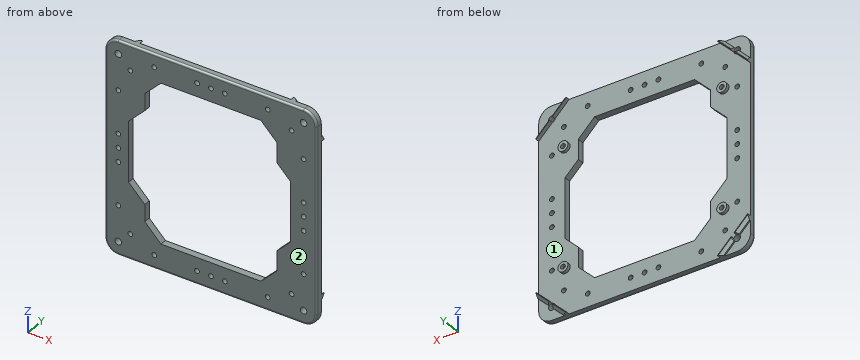
from build123d import *
from build123d.topology import SkipClean

# Parameters (mm, degrees)
SKETCH1_W           = 203.2
SKETCH1_H           = 203.2
BOSS_EXTRUDE1_DEPTH = 6.35
FILLET1_R           = 12.7
SKETCH2_R           = 3.175
CUT_EXTRUDE1_DEPTH  = 288.438345563
FILLET2_R           = 1.905
SKETCH3_R           = 2.286
CUT_EXTRUDE2_DEPTH  = 288.438345634
SKETCH4_R           = 2.286
CUT_EXTRUDE3_DEPTH  = 288.438345634
SKETCH5_R           = 4.826
SKETCH5_R_2         = 2.286
BOSS_EXTRUDE2_DEPTH = 3.175
BOSS_EXTRUDE3_DEPTH = 3.81
CHAMFER1_SIZE       = 2.54
CUT_EXTRUDE4_DEPTH  = 288.438345634
CHAMFER2_SIZE       = 15.5448
SKETCH8_R           = 2.286
CUT_EXTRUDE5_DEPTH  = 288.438345634


with BuildPart() as part:
    # Sketch1 → Boss-Extrude1 (new body)
    with BuildSketch(Plane(origin=(0, 0, 0), x_dir=(1, 0, 0), z_dir=(0, 1, 0))):
        with Locations((101.6, 101.6)):
            Rectangle(SKETCH1_W, SKETCH1_H)
    extrude(amount=BOSS_EXTRUDE1_DEPTH)

    # Fillet1
    fillet1_edges = [part.edges().sort_by_distance(p)[0] for p in [
        (0, 3.175, -203.2),
        (203.2, 3.175, -203.2),
        (203.2, 3.175, 0),
        (0, 3.175, 0),
    ]]
    fillet(fillet1_edges, radius=FILLET1_R)

    # Sketch2 → Cut-Extrude1 (cut, through all)
    with BuildSketch(Plane.XZ):
        with Locations(Location((12.7, -12.7, 0), (0, 0, 270))):
            Circle(SKETCH2_R)
        with Locations(Location((190.5, -12.7, 0), (0, 0, 270))):
            Circle(SKETCH2_R)
        with Locations(Location((190.5, -190.5, 0), (0, 0, 270))):
            Circle(SKETCH2_R)
        with Locations(Location((12.7, -190.5, 0), (0, 0, 270))):
            Circle(SKETCH2_R)
    extrude(amount=-CUT_EXTRUDE1_DEPTH, mode=Mode.SUBTRACT)

    # Fillet2
    fillet2_edges = [part.edges().sort_by_distance(p)[0] for p in [
        (0, 0, -101.6),
        (101.6, 0, -203.2),
        (203.2, 0, -101.6),
        (101.6, 0, 0),
        (199.480256121, 0, -199.480256121),
        (199.480256121, 0, -3.719743879),
        (3.719743879, 0, -3.719743879),
        (3.719743879, 0, -199.480256121),
    ]]
    fillet(fillet2_edges, radius=FILLET2_R)

    # Sketch3 → Cut-Extrude2 (cut, through all)
    with BuildSketch(Plane(origin=(0, 6.35, 0), x_dir=(1, 0, 0), z_dir=(0, 1, 0))):
        with Locations(Location((24.197781122, 24.197781122, 0), (0, 0, 270))):
            Circle(SKETCH3_R)
        with Locations(Location((179.002218878, 179.002218878, 0), (0, 0, 270))):
            Circle(SKETCH3_R)
        with Locations(Location((179.002218878, 24.197781122, 0), (0, 0, 270))):
            Circle(SKETCH3_R)
        with Locations(Location((24.197781122, 179.002218878, 0), (0, 0, 270))):
            Circle(SKETCH3_R)
    extrude(amount=-CUT_EXTRUDE2_DEPTH, mode=Mode.SUBTRACT)

    # Sketch4 → Cut-Extrude3 (cut, through all)
    with BuildSketch(Plane(origin=(0, 6.35, 0), x_dir=(1, 0, 0), z_dir=(0, 1, 0))):
        with Locations(Location((47.117, 12.7, 0), (0, 0, 270))):
            Circle(SKETCH4_R)
        with Locations(Location((156.083, 12.7, 0), (0, 0, 270))):
            Circle(SKETCH4_R)
        with Locations(Location((12.7, 156.083, 0), (0, 0, 270))):
            Circle(SKETCH4_R)
        with Locations(Location((12.7, 47.117, 0), (0, 0, 270))):
            Circle(SKETCH4_R)
        with Locations(Location((156.083, 190.5, 0), (0, 0, 270))):
            Circle(SKETCH4_R)
        with Locations(Location((47.117, 190.5, 0), (0, 0, 270))):
            Circle(SKETCH4_R)
        with Locations(Location((190.5, 47.117, 0), (0, 0, 270))):
            Circle(SKETCH4_R)
        with Locations(Location((190.5, 156.083, 0), (0, 0, 270))):
            Circle(SKETCH4_R)
        with Locations(Location((101.6, 12.7, 0), (0, 0, 270))):
            Circle(SKETCH4_R)
        with Locations(Location((12.7, 101.6, 0), (0, 0, 270))):
            Circle(SKETCH4_R)
        with Locations(Location((101.6, 190.5, 0), (0, 0, 270))):
            Circle(SKETCH4_R)
        with Locations(Location((190.5, 101.6, 0), (0, 0, 270))):
            Circle(SKETCH4_R)
    extrude(amount=-CUT_EXTRUDE3_DEPTH, mode=Mode.SUBTRACT)

    # Sketch5 → Boss-Extrude2 (add)
    # profile 1 of 4: a face of its own
    with BuildSketch(Plane(origin=(0, 6.35, 0), x_dir=(1, 0, 0), z_dir=(0, 1, 0))):
        with Locations(Location((25.4, 158.75, 0), (0, 0, 90))):
            Circle(SKETCH5_R)
        with Locations(Location((25.4, 158.75, 0), (0, 0, 270))):
            Circle(SKETCH5_R_2, mode=Mode.SUBTRACT)
    # profile 2 of 4: a face of its own
    with BuildSketch(Plane(origin=(0, 6.35, 0), x_dir=(1, 0, 0), z_dir=(0, 1, 0))):
        with Locations(Location((177.8, 158.75, 0), (0, 0, 90))):
            Circle(SKETCH5_R)
        with Locations(Location((177.8, 158.75, 0), (0, 0, 270))):
            Circle(SKETCH5_R_2, mode=Mode.SUBTRACT)
    # profile 3 of 4: a face of its own
    with BuildSketch(Plane(origin=(0, 6.35, 0), x_dir=(1, 0, 0), z_dir=(0, 1, 0))):
        with Locations(Location((177.8, 44.45, 0), (0, 0, 90))):
            Circle(SKETCH5_R)
        with Locations(Location((177.8, 44.45, 0), (0, 0, 270))):
            Circle(SKETCH5_R_2, mode=Mode.SUBTRACT)
    # profile 4 of 4: a face of its own
    with BuildSketch(Plane(origin=(0, 6.35, 0), x_dir=(1, 0, 0), z_dir=(0, 1, 0))):
        with Locations(Location((25.4, 44.45, 0), (0, 0, 90))):
            Circle(SKETCH5_R)
        with Locations(Location((25.4, 44.45, 0), (0, 0, 270))):
            Circle(SKETCH5_R_2, mode=Mode.SUBTRACT)
    extrude(amount=BOSS_EXTRUDE2_DEPTH)

    # Sketch6 → Boss-Extrude3 (add)
    with SkipClean():  # the faces are left unmerged after this step: merging them gives an invalid solid
        with BuildSketch(Plane(origin=(0, 6.35, 0), x_dir=(1, 0, 0), z_dir=(0, 1, 0))):
            with BuildLine():
                Line((203.2, 29.12872), (189.886429467, 15.815149467))
                ThreePointArc((189.886429467, 15.815149467), (191.679620112, 15.647731567), (193.093253903, 14.531845843))
                Line((193.093253903, 14.531845843), (203.2, 24.638591939))
                Line((203.2, 24.638591939), (203.2, 29.12872))
            make_face()
            with BuildLine():
                Line((178.561408061, 0), (174.07128, 0))
                Line((174.07128, 0), (187.384850533, 13.313570533))
                ThreePointArc((187.384850533, 13.313570533), (187.552268433, 11.520379888), (188.668154157, 10.106746097))
                Line((188.668154157, 10.106746097), (178.561408061, 0))
            make_face()
            with BuildLine():
                Line((13.313570533, 15.815149467), (0, 29.12872))
                Line((0, 29.12872), (0, 24.638591939))
                Line((0, 24.638591939), (10.106746097, 14.531845843))
                ThreePointArc((10.106746097, 14.531845843), (11.520379888, 15.647731567), (13.313570533, 15.815149467))
            make_face()
            with BuildLine():
                Line((24.638591939, 0), (14.531845843, 10.106746097))
                ThreePointArc((14.531845843, 10.106746097), (15.647731567, 11.520379888), (15.815149467, 13.313570533))
                Line((15.815149467, 13.313570533), (29.12872, 0))
                Line((29.12872, 0), (24.638591939, 0))
            make_face()
            with BuildLine():
                Line((15.815149467, 189.886429467), (29.12872, 203.2))
                Line((29.12872, 203.2), (24.638591939, 203.2))
                Line((24.638591939, 203.2), (14.531845843, 193.093253903))
                ThreePointArc((14.531845843, 193.093253903), (15.647731567, 191.679620112), (15.815149467, 189.886429467))
            make_face()
            with BuildLine():
                Line((0, 178.561408061), (10.106746097, 188.668154157))
                ThreePointArc((10.106746097, 188.668154157), (11.520379888, 187.552268433), (13.313570533, 187.384850533))
                Line((13.313570533, 187.384850533), (0, 174.07128))
                Line((0, 174.07128), (0, 178.561408061))
            make_face()
            with BuildLine():
                Line((189.886429467, 187.384850533), (203.2, 174.07128))
                Line((203.2, 174.07128), (203.2, 178.561408061))
                Line((203.2, 178.561408061), (193.093253903, 188.668154157))
                ThreePointArc((193.093253903, 188.668154157), (191.679620112, 187.552268433), (189.886429467, 187.384850533))
            make_face()
            with BuildLine():
                Line((178.561408061, 203.2), (188.668154157, 193.093253903))
                ThreePointArc((188.668154157, 193.093253903), (187.552268433, 191.679620112), (187.384850533, 189.886429467))
                Line((187.384850533, 189.886429467), (174.07128, 203.2))
                Line((174.07128, 203.2), (178.561408061, 203.2))
            make_face()
        extrude(amount=BOSS_EXTRUDE3_DEPTH)

    # Chamfer1
    chamfer1_edges = [part.edges().sort_by_distance(p)[0] for p in [
        (198.146626952, 10.16, -19.585218891),
        (183.614781109, 10.16, -5.053373048),
        (19.585218891, 10.16, -5.053373048),
        (5.053373048, 10.16, -19.585218891),
        (5.053373048, 10.16, -183.614781109),
        (19.585218891, 10.16, -198.146626952),
        (183.614781109, 10.16, -198.146626952),
        (198.146626952, 10.16, -183.614781109),
    ]]
    chamfer(chamfer1_edges, length=CHAMFER1_SIZE)

    # Sketch7 → Cut-Extrude4 (cut, through all)
    with BuildSketch(Plane(origin=(0, 6.35, 0), x_dir=(1, 0, 0), z_dir=(0, 1, 0))):
        Polygon((38.1, 57.15), (38.1, 25.4), (165.1, 25.4), (165.1, 57.15), (177.8, 57.15), (177.8, 146.05), (165.1, 146.05), (165.1, 177.8), (38.1, 177.8), (38.1, 146.05), (22.56850138, 146.05), (22.56850138, 57.15), align=None)
    extrude(amount=-CUT_EXTRUDE4_DEPTH, mode=Mode.SUBTRACT)

    # Chamfer2
    # the kernel refuses this chamfer: 15.5448 mm, written as the material it adds along each edge
    with BuildSketch(Plane(origin=(22.56850138, 6.35, -57.15), x_dir=(-0.027495876610586303, 0, -0.9996219169112966), z_dir=(0, -1, 0))) as chamfer2_piece_1_section:
        Polygon((CHAMFER2_SIZE * 0.999621916911, CHAMFER2_SIZE * 0.0274958766106), (-CHAMFER2_SIZE * 0.0274958766106, CHAMFER2_SIZE * 0.999621916911), (0, 0), align=None)
    chamfer2_piece_1 = extrude(amount=6.35, mode=Mode.PRIVATE)
    chamfer2_piece_1 = split(chamfer2_piece_1, bisect_by=Plane(origin=(38.1, 3.175, -62.286463207), z_dir=(-1, 0, 0)), keep=Keep.TOP, mode=Mode.PRIVATE)
    add(chamfer2_piece_1)
    with BuildSketch(Plane(origin=(38.1, 6.35, -25.4), x_dir=(-0.027495876610586754, 0, -0.9996219169112966), z_dir=(0, -1, 0)), Plane(origin=(165.1, 6.35, -25.4), x_dir=(-0.9996219169112966, 0, 0.027495876610586292), z_dir=(0, -1, 0)), Plane(origin=(165.1, 6.35, -177.8), x_dir=(0.027495876610586292, 0, 0.9996219169112966), z_dir=(0, -1, 0)), Plane(origin=(38.1, 6.35, -177.8), x_dir=(0.9996219169112966, 0, -0.027495876610586317), z_dir=(0, -1, 0))) as chamfer2_piece_2:
        Polygon((CHAMFER2_SIZE * 0.999621916911, CHAMFER2_SIZE * 0.0274958766106), (-CHAMFER2_SIZE * 0.0274958766106, CHAMFER2_SIZE * 0.999621916911), (0, 0), align=None)
    extrude(amount=6.35)
    with BuildSketch(Plane(origin=(177.8, 6.35, -57.15), x_dir=(-0.9996219169112966, 0, 0.027495876610586292), z_dir=(0, -1, 0))) as chamfer2_piece_3_section:
        Polygon((CHAMFER2_SIZE * 0.999621916911, CHAMFER2_SIZE * 0.0274958766106), (-CHAMFER2_SIZE * 0.0274958766106, CHAMFER2_SIZE * 0.999621916911), (0, 0), align=None)
    chamfer2_piece_3 = extrude(amount=6.35, mode=Mode.PRIVATE)
    chamfer2_piece_3 = split(chamfer2_piece_3, bisect_by=Plane(origin=(165.1, 3.175, -62.494102003), z_dir=(1, 0, 0)), keep=Keep.TOP, mode=Mode.PRIVATE)
    add(chamfer2_piece_3)
    with BuildSketch(Plane(origin=(177.8, 6.35, -146.05), x_dir=(0.027495876610586292, 0, 0.9996219169112966), z_dir=(0, -1, 0))) as chamfer2_piece_4_section:
        Polygon((CHAMFER2_SIZE * 0.999621916911, CHAMFER2_SIZE * 0.0274958766106), (-CHAMFER2_SIZE * 0.0274958766106, CHAMFER2_SIZE * 0.999621916911), (0, 0), align=None)
    chamfer2_piece_4 = extrude(amount=6.35, mode=Mode.PRIVATE)
    chamfer2_piece_4 = split(chamfer2_piece_4, bisect_by=Plane(origin=(165.1, 3.175, -140.705897997), z_dir=(1, 0, 0)), keep=Keep.TOP, mode=Mode.PRIVATE)
    add(chamfer2_piece_4)
    with BuildSketch(Plane(origin=(22.56850138, 6.35, -146.05), x_dir=(0.9996219169112966, 0, -0.027495876610586303), z_dir=(0, -1, 0))) as chamfer2_piece_5_section:
        Polygon((CHAMFER2_SIZE * 0.999621916911, CHAMFER2_SIZE * 0.0274958766106), (-CHAMFER2_SIZE * 0.0274958766106, CHAMFER2_SIZE * 0.999621916911), (0, 0), align=None)
    chamfer2_piece_5 = extrude(amount=6.35, mode=Mode.PRIVATE)
    chamfer2_piece_5 = split(chamfer2_piece_5, bisect_by=Plane(origin=(38.1, 3.175, -140.913536793), z_dir=(-1, 0, 0)), keep=Keep.TOP, mode=Mode.PRIVATE)
    add(chamfer2_piece_5)

    # Sketch8 → Cut-Extrude5 (cut, through all)
    with BuildSketch(Plane(origin=(0, 6.35, 0), x_dir=(1, 0, 0), z_dir=(0, 1, 0))):
        with Locations(Location((88.265, 12.7, 0), (0, 0, 270))):
            Circle(SKETCH8_R)
        with Locations(Location((114.935, 12.7, 0), (0, 0, 270))):
            Circle(SKETCH8_R)
        with Locations(Location((101.6, 12.7, 0), (0, 0, 270))):
            Circle(SKETCH8_R)
        with Locations(Location((12.7, 114.935, 0), (0, 0, 270))):
            Circle(SKETCH8_R)
        with Locations(Location((12.7, 88.265, 0), (0, 0, 270))):
            Circle(SKETCH8_R)
        with Locations(Location((114.935, 190.5, 0), (0, 0, 270))):
            Circle(SKETCH8_R)
        with Locations(Location((88.265, 190.5, 0), (0, 0, 270))):
            Circle(SKETCH8_R)
        with Locations(Location((190.5, 88.265, 0), (0, 0, 270))):
            Circle(SKETCH8_R)
        with Locations(Location((190.5, 114.935, 0), (0, 0, 270))):
            Circle(SKETCH8_R)
    extrude(amount=-CUT_EXTRUDE5_DEPTH, mode=Mode.SUBTRACT)


solid = part.part
Read the model definition and answer for the solid it produces. Units are mm, in the model's axes. Face numbers are marked on the shaded views. Round coordinates to 2 decimals unless told otherwise and drop trailing zeros. Write each loop counter-clockwise with the first axis right and the second up, starting at its lowest first coordinate (ties: lowest second). Pieces come first, ordered by that corner, then holes.
1. Given pin 1 Ø5.5 at (x, z) = (190.5, -190.5) entering from -Y; pin 2 Ø7.5 at (x, z) = (179, -24.2) entering from +Y; pin 3 Ø5 at (x, z) = (25, -45.5) entering from +Y (3 decimals), each flat-ended and moving along its own axis, determine where each tip first touches the part or whether it passes through.
2. Determine the mould class of the marked faces 1 and 2 for opening direction Z: pulls with the +Z half, pulls with the -Z half, needs draft (parallel to the pull), parting line crosses it, or undercut.
3. The part is cut by section B-B, the plane y = 3.75. State how many separate pieces and enclosed holes the cut face has, then the cut area to 3 significant figures.
4. Straight lines are drawn through the part: L1, parallel to X at y = 2.5, z = -102; L2, parallel to Z at x = 55, y = 6.25; L3, parallel to Z at x = 47.5, y = 6. For each, find the intervals that lie inside material, in ascending order.
5. The part is cut by section A-A, the plane z = -33. Determine the outline of the cut face in (x, y) (3 decimals).
Values:
1. pin 1: passes through
1. pin 2: stops at y = 6.35
1. pin 3: stops at y = 9.525
2. face 1: undercut
2. face 2: needs draft
3. separate pieces: 1
3. enclosed holes: 29
3. area: 19,700 mm2
4. L1: x = 0 to 10.45, 14.95 to 22.57, 177.8 to 188.25, 192.75 to 203.2
4. L2: z = -203.2 to -177.8, -25.4 to 0
4. L3: z = -203.2 to -192.75, -188.25 to -171.66, -31.54 to -14.95, -10.45 to 0
5. outline: (0, 1.905) arc R1.905 ccw to (1.905, 0) - (46.045, 0) - (46.045, 6.35) - (0, 6.35) - close; (157.155, 0) - (201.295, 0) arc R1.905 ccw to (203.2, 1.905) - (203.2, 6.35) - (157.155, 6.35) - close
